For this review, take the finished solid that the model builds, in its own axes (mm). Face numbers are marked on the shaded views. A direction names the side the tool comes from. Coordinates: 2 decimals unless noted, no trailing zeros. Order: outer loops, then holes, each group sorted by start corner. A loop starts at its lowest first (then second) coordinate and runs counter-clockwise, first axis right, second up.
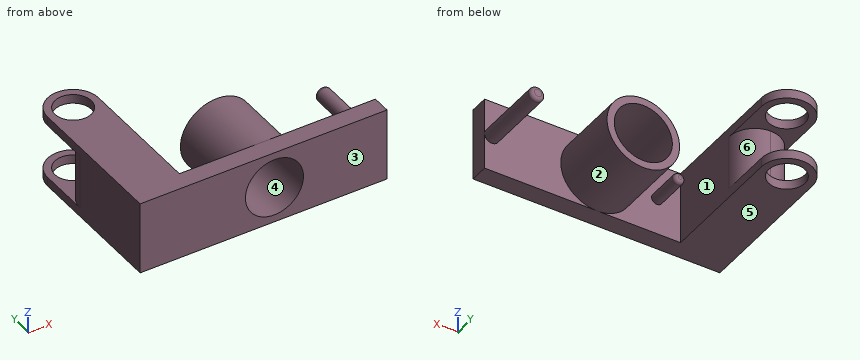
Autodesk Inventor part; units mm, degrees
ref_plane "YZ Plane" through (0, 0, 0) normal (1, 0, 0) x (0, 1, 0)
ref_plane "XZ Plane" through (0, 0, 0) normal (0, 1, 0) x (-1, 0, 0)
ref_plane "XY Plane" through (0, 0, 0) normal (0, 0, 1) x (1, 0, 0)
sketch "Sketch1" plane through (0, 0, 0) normal (0, 0, 1) x (1, 0, 0)
  line L0 (0, 0) -> (0, 40)
  line L1 (0, 0) -> (68, 0)
  line L2 (68, 0) -> (68, 5)
  line L3 (68, 5) -> (14, 5)
  arc A0 (14, 40) -> (0, 40) centre (7, 40) ccw
  line L4 (14, 40) -> (14, 5)
  circle A1 centre (7, 40) radius 5
  dimension "d0" = 40
  dimension "d2" = 5
  dimension "d6" = 7
  dimension "d7" = 10
  dimension "d8" = 14
  dimension "d9" = 54
extrude "Extrusion1" add sketch "Sketch1" along normal blind 20
sketch "Sketch2" plane through (14, 5, 0) normal (0, 1, 0) x (1, 0, 0)
  circle A0 centre (6.5, -10) radius 1.5
  line L0 (0, 0) -> (0, -20)
  circle A1 centre (23, -10) radius 10
  line L1 (0, 0) -> (54, 0)
  circle A2 centre (52, -10) radius 2
  line L2 (54, 0) -> (54, -20)
  point P0 (-14, 0)
  dimension "d12" = 3
  dimension "d13" = 6.5
  dimension "d14" = 20
  dimension "d16" = 23
  dimension "d19" = 10
  dimension "d20" = 4
  dimension "d21" = 10
  dimension "d22" = 17
extrude "Extrusion2" add sketch "Sketch2" along normal blind 20
sketch "Sketch4" plane through (0, 0, 20) normal (0, 0, 1) x (1, 0, 0)
  line L0 (22, 25) -> (19, 25)
  line L1 (19, 25) -> (22, 25)
  line L2 (22, 5) -> (22, 25)
  line L3 (22, 25) -> (22, 15)
  line L4 (22, 15) -> (19, 15)
  line L5 (19, 5) -> (19, 25)
  point P0 (0, 0)
  dimension "d25" = 10
extrude "Extrusion3" cut sketch "Sketch4" against normal blind 20
fillet "Fillet1" radius 1 1 edges at (19, 15, 10)
fillet "Fillet2" radius 1 1 edges at (64, 25, 10)
sketch "Sketch5" plane through (37, 25, 10) normal (0, 1, 0) x (1, 0, 0)
  circle A0 centre (0, 0) radius 8
  point P0 (-37, 10)
  dimension "d30" = 16
extrude "Extrusion4" cut sketch "Sketch5" against normal blind 30
sketch "Sketch6" plane through (14, 5, 0) normal (1, 0, 0) x (0, 0, -1)
  point P0 (0, -5)
sketch "Sketch7" plane through (14, 5, 0) normal (1, 0, 0) x (0, 0, -1)
  line L0 (-10, 41.0364) -> (-10, 39.6436)
  line L1 (0, 42) -> (-20, 42)
  line L2 (-2.5, 42) -> (-2.5, 28)
  line L3 (-17.5, 42) -> (-17.5, 28)
  line L4 (-17.5, 42) -> (-2.5, 42)
  line L5 (0, 30) -> (-20, 30)
  line L6 (-17.5, 28) -> (-2.5, 28)
  point P0 (0, -5)
  dimension "d40" = 14
  dimension "d41" = 14
  dimension "d42" = 15
extrude "Extrusion5" cut sketch "Sketch7" against normal blind 14
fillet "Fillet3" radius 7 2 edges at (14, 33, 10) (0, 33, 10)
equation "\"d19\" = 0.5 * d14"
equation "\"d21\" = d19"
equation "\"d40\" = d41"
properties part number "ValveMk2"
1. Machinability: for the marked faces 1, 2 and 3, which of the approach directions +Z, -Z, +X, -X, +Y, -Y give a long, thin tool a straight path to every point of the face, cutting with its end or side? Answer none if there is none.
Answer below:
face 1: +Z, -Z, +Y
face 2: +Y
face 3: +Z, -Z, +X, -X, -Y
2. Take a section at A-A, the plane y = 16. Give the boundary of the cut face in (x, z), plus the area to 3 significant figures.
Answer below:
outline: (0, 0) - (14, 0) - (14, 20) - (0, 20) - close; circle Ø20 at (37, 10); circle Ø4 at (66, 10); hole circle Ø16 at (37, 10)
area: 406 mm2
3. The part is to be moulded in two halves that separate along X. For the marked faces 4, 5 and 6, say which applies: +X half, -X half, draft (parallel to the pull), parting line (faces both ways), or undercut.
Answer below:
face 4: undercut
face 5: draft
face 6: +X half
4. To check wall thickness, follow L1, parallel to X at y = 13.75, z = 10; L2, parallel to Y at x = 7, z = 1.35; L3, parallel to X at y = 40, z = 1.2. State the ranges of each line that lie inside material, in increasing order.
Answer below:
L1: x = 0 to 14, 19 to 22, 27 to 29, 45 to 47, 64 to 68
L2: y = 0 to 35, 45 to 47
L3: x = 0 to 2, 12 to 14
5. Take a section at D-D, the plane y = 37.5. Give the boundary of the cut face in (x, z).
Answer below:
outline: (0, 0) - (2.67, 0) - (2.67, 2.5) - (0, 2.5) - close; (0, 17.5) - (2.67, 17.5) - (2.67, 20) - (0, 20) - close; (11.33, 0) - (14, 0) - (14, 2.5) - (11.33, 2.5) - close; (11.33, 17.5) - (14, 17.5) - (14, 20) - (11.33, 20) - close
6. Take a section at B-B, the plane x = 5.5. Give the boundary of the cut face in (y, z), plus the area to 3 significant figures.
Answer below:
outline: (0, 0) - (35.23, 0) - (35.23, 2.5) - (32.84, 2.5) - (32.84, 17.5) - (35.23, 17.5) - (35.23, 20) - (0, 20) - close; (44.77, 0) - (46.84, 0) - (46.84, 2.5) - (44.77, 2.5) - close; (44.77, 17.5) - (46.84, 17.5) - (46.84, 20) - (44.77, 20) - close
area: 679 mm2
7. Clearance check with flat-ended pins moving along their axes: pin 1 Ø1.5 at (y, z) = (35, 5.5) entering from +X; pin 2 Ø1.1 at (x, z) = (20.5, 10) entering from +Y; pin 3 Ø10 at (y, z) = (29, 15.5) entering from +X; pin 4 Ø4 at (x, y) = (28, 10.5) entering from +Z. State where each tip first meets the part, or that it passes through.
Answer below:
pin 1: passes through
pin 2: stops at y = 15
pin 3: stops at x = 46.68
pin 4: stops at z = 17.14
